For this review, use the dimensioned drawing (mm, ordinates from the lowest corner) and the shaded views. Give positions to 0.01 mm unless a question says otherwise; leave off trailing zeros. Loops run counter-clockwise (first coordinate to the right, second up) from the corner with the lowest first, then second, coordinate; pieces in that order, holes last. Notation, with made-up numbers: (-31.75, 89) -> (-23.75, 89) arc R32 cw to (-23.75, 127) -> close; hole circle Ø7 at (76.25, 24). An arc over 180 degrees is marked (long way). Use a Markdown table: item, result. Add a question column.
1. Add section C-C (z = 0.4). State the section outline as (x, y) points, and give its area (3 significant figures).
2. Add section A-A (x = 4). State the section outline as (y, z) points, and give its area (3 significant figures).
3. Add section D-D (x = 2.25). State the section outline as (y, z) points.
4. To check wall thickness, follow line 1 (Y direction, x = 4, z = 0.85); line 2 (X direction, y = 5.25, z = 0.85); line 3 (X direction, y = 5, z = 0.3). State the ranges of each line that lie inside material, in increasing order.
5. Draft analysis for pull direction X (two halves, no side actions). For the marked faces 1, 2 and 3, state which applies: pulls with the +X half, pulls with the -X half, needs draft (parallel to the pull), parting line crosses it, or undercut.
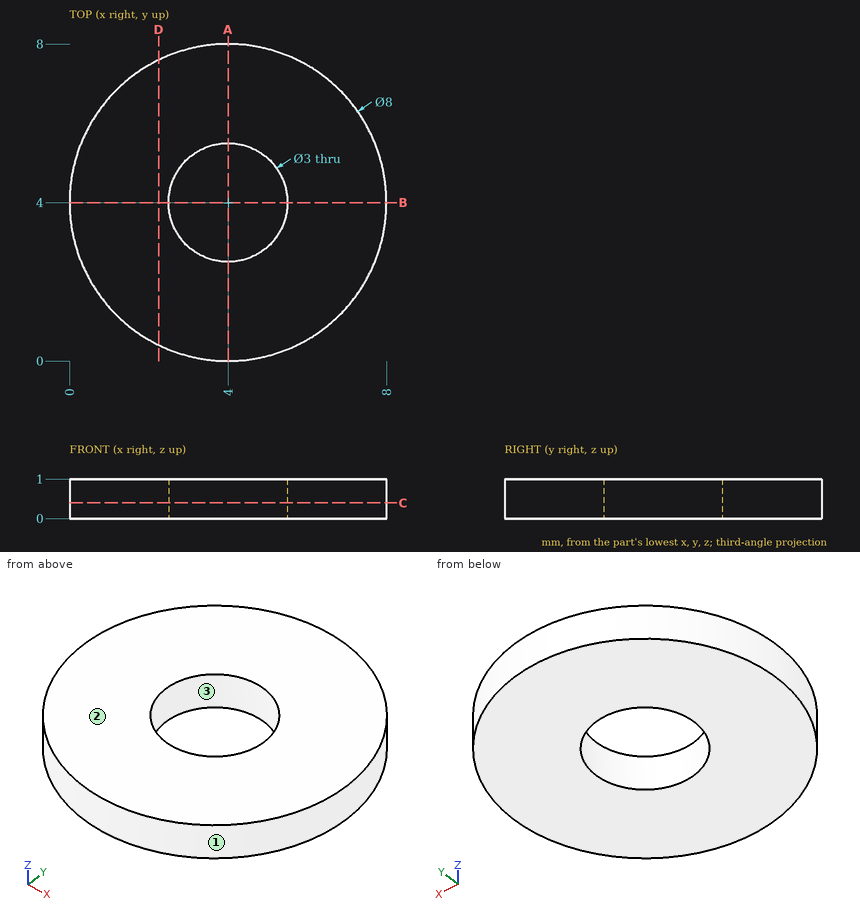
Taken from the geometry:
| question | item | result |
|---|---|---|
| 1 | outline | circle Ø8 at (4, 4); hole circle Ø3 at (4, 4) |
| 1 | area | 43.2 mm^2 |
| 2 | outline | (0, 0) -> (2.5, 0) -> (2.5, 1) -> (0, 1) -> close; (5.5, 0) -> (8, 0) -> (8, 1) -> (5.5, 1) -> close |
| 2 | area | 5.00 mm^2 |
| 3 | outline | (0.4, 0) -> (7.6, 0) -> (7.6, 1) -> (0.4, 1) -> close |
| 4 | line 1 | y = 0 to 2.5, 5.5 to 8 |
| 4 | line 2 | x = 0.2 to 3.17, 4.83 to 7.8 |
| 4 | line 3 | x = 0.13 to 2.88, 5.12 to 7.87 |
| 5 | face 1 | parting line crosses it |
| 5 | face 2 | needs draft |
| 5 | face 3 | undercut |
